Autodesk Inventor part; units mm, degrees
ref_plane "YZ Plane" through (0, 0, 0) normal (1, 0, 0) x (0, 1, 0)
ref_plane "XZ Plane" through (0, 0, 0) normal (0, 1, 0) x (-1, 0, 0)
ref_plane "XY Plane" through (0, 0, 0) normal (0, 0, 1) x (1, 0, 0)
sketch "Sketch1" plane through (0, 0, 0) normal (0, 0, 1) x (1, 0, 0)
  circle A0 centre (0, 0) radius 34
  circle A1 centre (0, 0) radius 9
  circle A2 centre (0, 28.25) radius 5
  circle A3 centre (-28.25, 0) radius 5
  circle A4 centre (0, -28.25) radius 5
  circle A5 centre (28.25, 0) radius 5
  arc A6 (4.9804, 27.8075) -> (-4.9804, 27.8075) centre (0, 0) ccw
  arc A7 (27.8075, -4.9804) -> (27.8075, 4.9804) centre (0, 0) ccw
  arc A8 (-27.8075, 4.9804) -> (-27.8075, -4.9804) centre (0, 0) ccw
  arc A9 (-4.9804, -27.8075) -> (4.9804, -27.8075) centre (0, 0) ccw
  dimension "d0" = 68
  dimension "d1" = 18
  dimension "d3" = 10
  dimension "d6" = 360
extrude "Extrusion1" add sketch "Sketch1" along normal blind 2
properties part number "Black Rubber Pad Bottom"
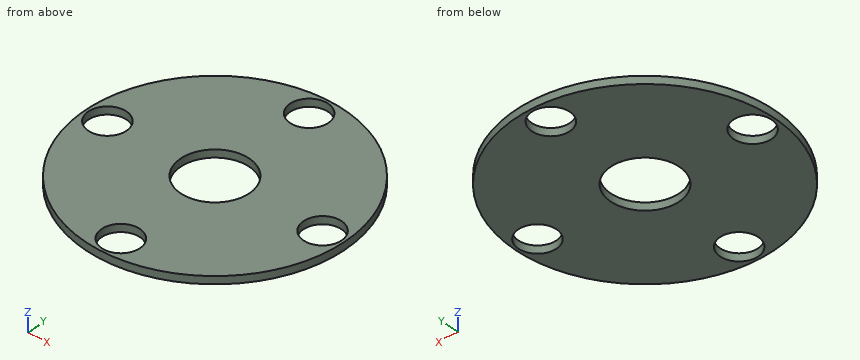
The listing builds one solid part. Answer for the finished solid, in the listing's coordinates (mm). Give positions to 0.01 mm unless a question says otherwise; leave off trailing zeros. Write each loop counter-clockwise with the first axis right and the second up, starting at its lowest first coordinate (ties: lowest second). Pieces come first, ordered by that corner, then holes. Notation, with made-up numbers: (-15, 62.5) - (41, 62.5) arc R23 ccw to (41, 74.5) - close; hole circle Ø2 at (85.25, 62.5). An arc over 180 degrees is marked (long way). Use a Markdown table: item, result.
1. Section A-A on y = 0 is taken. Write down the section's boundary in (x, z), plus the area to 3 significant figures.
Values follow:
| item | result |
|---|---|
| outline | (-34, 0) - (-33.25, 0) - (-33.25, 2) - (-34, 2) - close; (-23.25, 0) - (-9, 0) - (-9, 2) - (-23.25, 2) - close; (9, 0) - (23.25, 0) - (23.25, 2) - (9, 2) - close; (33.25, 0) - (34, 0) - (34, 2) - (33.25, 2) - close |
| area | 60.0 mm² |
2. Section B-B on z = 1.7 is taken. Write down the section's boundary in (x, y), plus the area to 3 significant figures.
Values follow:
| item | result |
|---|---|
| outline | circle Ø68 at (0, 0); hole circle Ø10 at (-28.25, 0); hole circle Ø18 at (0, 0); hole circle Ø10 at (0, -28.25); hole circle Ø10 at (0, 28.25); hole circle Ø10 at (28.25, 0) |
| area | 3,060 mm² |
3. Each of these flat-tipped pins is pushed along its axis until it touches: P1, Ø9, axis at x = 0, y = 28.25, coming from the -Z side; P2, Ø1, axis at x = 3.5, z = 0.5, coming from the +Y side. Where does it stop, or does it pass through?
Values follow:
| item | result |
|---|---|
| P1 | passes through |
| P2 | stops at y = 33.87 |
4. Section D-D on y = -28.25 is taken. Write down the section's boundary in (x, z), plus the area to 3 significant figures.
Values follow:
| item | result |
|---|---|
| outline | (-18.92, 0) - (-5, 0) - (-5, 2) - (-18.92, 2) - close; (5, 0) - (18.92, 0) - (18.92, 2) - (5, 2) - close |
| area | 55.7 mm² |
5. Find the intervals of material crossed by probe 1 along Y at (x, z) = (0, 1.4); probe 2 along X at (y, z) = (-25.5, 1.6); probe 3 along Y at (x, z) = (-28.25, 0.9), in increasing order. Write a range as from..to.
Values follow:
| item | result |
|---|---|
| probe 1 | y = -34..-33.25, -23.25..-9, 9..23.25, 33.25..34 |
| probe 2 | x = -22.49..-4.18, 4.18..22.49 |
| probe 3 | y = -18.92..-5, 5..18.92 |
6. Section C-C on x = -28 is taken. Write down the section's boundary in (y, z).
Values follow:
| item | result |
|---|---|
| outline | (-19.29, 0) - (-4.99, 0) - (-4.99, 2) - (-19.29, 2) - close; (4.99, 0) - (19.29, 0) - (19.29, 2) - (4.99, 2) - close |
